from build123d import *

# Parameters (mm, degrees)
BOSS_EXTRUDE1_DEPTH = 2.8
SKETCH2_W           = 5.05
SKETCH2_H           = 1.4
BOSS_EXTRUDE2_DEPTH = 0.1
FILLET1_R           = 0.1


with BuildPart() as part:
    # Sketch1 → Boss-Extrude1 (new body)
    with BuildSketch(Plane.XY):
        with BuildLine():
            Line((-2.9, -3.2), (2.9, -3.2))
            ThreePointArc((2.9, -3.2), (3.253553391, -3.053553391), (3.4, -2.7))
            Line((3.4, -2.7), (3.4, 2.7))
            ThreePointArc((3.4, 2.7), (3.253553391, 3.053553391), (2.9, 3.2))
            Line((2.9, 3.2), (-2.9, 3.2))
            ThreePointArc((-2.9, 3.2), (-3.253553391, 3.053553391), (-3.4, 2.7))
            Line((-3.4, 2.7), (-3.4, -2.7))
            ThreePointArc((-3.4, -2.7), (-3.253553391, -3.053553391), (-2.9, -3.2))
        make_face()
    extrude(amount=BOSS_EXTRUDE1_DEPTH)

    # Sketch2 → Boss-Extrude2 (add)
    with BuildSketch(Plane(origin=(0, 0, 0), x_dir=(-1, 0, 0), z_dir=(0, 0, -1))):
        with Locations((0, 2)):
            Rectangle(SKETCH2_W, SKETCH2_H)
        with Locations((0, -2)):
            Rectangle(SKETCH2_W, SKETCH2_H)
    extrude(amount=BOSS_EXTRUDE2_DEPTH)

    # Fillet1
    fillet1_edges = [part.edges().sort_by_distance(p)[0] for p in [
        (3.253553391, 3.053553391, 2.8),
        (3.4, 0, 0),
        (3.253553391, -3.053553391, 0),
        (0, 3.2, 2.8),
        (-3.253553391, 3.053553391, 2.8),
        (-3.4, 0, 2.8),
        (-3.253553391, -3.053553391, 2.8),
        (0, -3.2, 2.8),
        (3.253553391, -3.053553391, 2.8),
        (3.4, 0, 2.8),
        (0, -3.2, 0),
        (-3.253553391, -3.053553391, 0),
        (-3.4, 0, 0),
        (-3.253553391, 3.053553391, 0),
        (0, 3.2, 0),
        (3.253553391, 3.053553391, 0),
    ]]
    fillet(fillet1_edges, radius=FILLET1_R)


solid = part.part
Geometry: final body of the model. Coordinates: model frame, mm. Give positions to 0.01 mm unless a question says otherwise; leave off trailing zeros. Write each loop counter-clockwise with the first axis right and the second up, starting at its lowest first coordinate (ties: lowest second). Pieces come first, ordered by that corner, then holes. Notation, with made-up numbers: (-36, -35) -> (8, -35) arc R19 cw to (8, -16) -> close; hole circle Ø2 at (73.25, 64.5). An arc over 180 degrees is marked (long way). Answer in a Markdown table with one row per item.
(1) Draft query along Y for faces 1 (the flat face through (0, -3.2, 1)), 2 (the flat face through (0, 3.2, 1)), 3 (the flat face through (0, 0, 0)), 4 (the flat face through (0, -2, -0.1)). Return one class per face: +Y half, -Y half, draft (parallel to the pull), parting line (faces both ways), or undercut.
Answers below:
| item | result |
|---|---|
| face 1 | -Y half |
| face 2 | +Y half |
| face 3 | undercut |
| face 4 | draft |
(2) Ray query, line 1 along Z through (x, y) = (-2.5, -0.5); line 2 along Y through (x, z) = (3, 1.1); line 3 along Y through (x, z) = (3.25, 0.15). Return the intervals inside material, ascending. Write a range as [from, to].
Answers below:
| item | result |
|---|---|
| line 1 | [0, 2.8] |
| line 2 | [-3.19, 3.19] |
| line 3 | [-3.06, 3.06] |
(3) Section query A-A on y = -1. Return loops of the section in (x, z), then the cut area to 3 significant figures.
Answers below:
| item | result |
|---|---|
| outline | (-3.4, 0.1) arc R0.1 ccw to (-3.3, 0) -> (3.3, 0) arc R0.1 ccw to (3.4, 0.1) -> (3.4, 2.7) arc R0.1 ccw to (3.3, 2.8) -> (-3.3, 2.8) arc R0.1 ccw to (-3.4, 2.7) -> close |
| area | 19.0 mm^2 |
(4) Section query B-B on x = 2.75. Return loops of the section in (y, z).
Answers below:
| item | result |
|---|---|
| outline | (-3.2, 0.1) arc R0.1 ccw to (-3.1, 0) -> (3.1, 0) arc R0.1 ccw to (3.2, 0.1) -> (3.2, 2.7) arc R0.1 ccw to (3.1, 2.8) -> (-3.1, 2.8) arc R0.1 ccw to (-3.2, 2.7) -> close |
